Could you check a few things on this model? Use its own coordinates, in mm. A direction names the side the tool comes from. Coordinates: 2 decimals unless noted, no trailing zeros. Write each loop counter-clockwise with the first axis right and the second up, starting at its lowest first coordinate (ties: lowest second). Pieces come first, ordered by that corner, then holes.
Item 1: I want a section at B-B on x = -6. Please give me the cut outline in (y, z), then the cut area to 3 significant figures.
Item 2: If I drill on probe 1 along Z at (x, y) = (-15.5, 7.5); probe 2 along X at (y, z) = (2, -18); probe 3 along Z at (x, y) = (11, 4.75), over which ranges is the centre line in solid material (lowest first)?
Item 3: For P1, Ø8, axis at x = -11.5, z = 4.5, coming from the +Y side; P2, Ø1.1, axis at x = 17.5, z = 2.5, coming from the +Y side; P3, Ø5, axis at x = -11.5, z = 18.5, coming from the -Y side, each with a flat end and sliding along its axis, tell me the tip position at first contact or that it passes through.
Item 4: Thinking about a two-plate mould opening in Z: for faces 4 (the flat face through (0, 4, 23.35)), 5 (the flat face through (0, 0, 0)), 6 (the cylindrical face through (-17.407, 5.403, -11.359)), which applies, +Z half, -Z half, draft (parallel to the pull), parting line (faces both ways), or undercut?
Item 5: I want a section at A-A on z = -5. Please give me the cut outline in (x, y), then the cut area to 3 significant figures.
Item 6: Which directions (+Z, -Z, +X, -X, +Y, -Y) give clear straight access to the entire face, cutting with the end or side of a thin tool? Please do faces 1 (the flat face through (-17.4, 4.2, -0.1)), 2 (the flat face through (11.5, 0.6, -21.35)), 3 (the flat face through (8.345, 4, -22)).
Item 7: I want a section at C-C on y = 7.5. Please give me the cut outline in (x, z) (3 decimals), then the cut area to 3 significant figures.
Autodesk Inventor part; units mm, degrees
ref_plane "YZ Plane" through (0, 0, 0) normal (1, 0, 0) x (0, 1, 0)
ref_plane "XZ Plane" through (0, 0, 0) normal (0, 1, 0) x (-1, 0, 0)
ref_plane "XY Plane" through (0, 0, 0) normal (0, 0, 1) x (1, 0, 0)
sketch "Sketch1" plane through (0, 0, 0) normal (0, 1, 0) x (-1, 0, 0)
  line L0 (17.9, -23.35) -> (-17.9, -23.35)
  line L1 (-17.9, -23.35) -> (-17.9, 23.35)
  line L2 (-17.9, 23.35) -> (17.9, 23.35)
  line L3 (17.9, 23.35) -> (17.9, -23.35)
  point P0 (0, 0)
  dimension "d0" = 35.8
  dimension "d1" = 46.7
  dimension "d2" = 23.35
  dimension "d3" = 17.9
extrude "Extrusion1" add sketch "Sketch1" along normal blind 8.2
sketch "Sketch2" plane through (0, 8.2, 0) normal (0, 1, 0) x (1, 0, 0)
  line L0 (-16.8, -22.25) -> (16.8, -22.25)
  line L1 (16.8, -22.25) -> (16.8, 21.35)
  line L2 (16.8, 21.35) -> (-16.8, 21.35)
  line L3 (-16.8, 21.35) -> (-16.8, -22.25)
  line L4 (-17.9, -23.35) -> (17.9, -23.35)
  line L5 (17.9, -23.35) -> (17.9, 23.35)
  line L6 (-17.9, 23.35) -> (-17.9, -23.35)
  line L7 (17.9, 23.35) -> (-17.9, 23.35)
  point P0 (0, 0)
  dimension "d6" = 1.1
  dimension "d7" = 1.1
  dimension "d8" = 1.1
  dimension "d9" = 2
extrude "Extrusion2" cut sketch "Sketch2" against normal blind 7.1 contours L3 L2 L1 L0
sketch "Sketch6" plane through (17.9, 0, 23.35) normal (1, 0, 0) x (0, 0, -1)
  line L0 (1.1, 8.2) -> (44.7, 8.2)
  line L1 (10.85, 8.2) -> (35.85, 8.2)
  line L2 (35.85, 8.2) -> (35.85, 4.2)
  line L3 (35.85, 4.2) -> (10.85, 4.2)
  line L4 (10.85, 4.2) -> (10.85, 8.2)
  line L5 (46.7, 0) -> (46.7, 8.2)
  point P0 (23.35, 0)
  dimension "d34" = 25
  dimension "d35" = 10.85
  dimension "d36" = 4
extrude "Extrusion6" cut sketch "Sketch6" against normal through all
fillet "Fillet2" radius 4 4 edges at (17.35, 4.2, 12.5) (-17.35, 4.2, 12.5) (-17.35, 4.2, -12.5) (17.35, 4.2, -12.5)
sketch "Sketch9" plane through (0, 8.2, 0) normal (0, 1, 0) x (1, 0, 0)
  point P0 (0, 0)
sketch "Sketch10" plane through (0, 8.2, 0) normal (0, 1, 0) x (1, 0, 0)
  line L0 (-16.8, 21.35) -> (16.8, 21.35)
  line L1 (12.55, 21.35) -> (10.55, 21.35)
  line L2 (10.55, 21.35) -> (10.55, 22.35)
  line L3 (10.55, 22.35) -> (12.55, 22.35)
  line L4 (12.55, 22.35) -> (12.55, 21.35)
  line L5 (8.345, 21.35) -> (6.345, 21.35)
  line L6 (6.345, 21.35) -> (6.345, 22.35)
  line L7 (6.345, 22.35) -> (8.345, 22.35)
  line L8 (8.345, 22.35) -> (8.345, 21.35)
  line L9 (17.9, 23.35) -> (-17.9, 23.35)
  line L10 (17.9, 12.5) -> (17.9, 23.35)
  point P0 (0, 0)
  dimension "d51" = 2
  dimension "d52" = 2
  dimension "d53" = 2.205
  dimension "d54" = 1
  dimension "d55" = 5.35
extrude "Extrusion9" cut sketch "Sketch10" against normal through all
sketch "Sketch12" plane through (0, 8.2, 0) normal (0, 1, 0) x (1, 0, 0)
  line L0 (6.345, 22.35) -> (8.345, 22.35)
  line L1 (6.345, 22.35) -> (8.345, 22.35)
  line L2 (8.345, 22.35) -> (8.345, 22.649)
  line L3 (8.345, 22.649) -> (6.345, 22.649)
  line L4 (6.345, 22.649) -> (6.345, 22.35)
  line L5 (10.55, 22.35) -> (12.55, 22.35)
  line L6 (10.55, 22.35) -> (12.5613, 22.35)
  line L7 (12.5613, 22.35) -> (12.5613, 22.649)
  line L8 (12.5613, 22.649) -> (10.55, 22.649)
  line L9 (10.55, 22.649) -> (10.55, 22.35)
  point P0 (0, 0)
extrude "Extrusion11" cut sketch "Sketch12" against normal through all
sketch "Sketch13" plane through (17.9, 0, -23.35) normal (0, 0, -1) x (-1, 0, 0)
  line L0 (7.35, 0) -> (5.35, 0)
  line L1 (7.35, 8.2) -> (7.35, 1.1)
  line L2 (5.35, 0) -> (7.35, 0)
  line L3 (7.35, 0) -> (7.35, 2.5)
  line L4 (7.35, 2.5) -> (5.35, 2.5)
  line L5 (5.35, 2.5) -> (5.35, 0)
  line L6 (11.555, 0) -> (9.555, 0)
  line L7 (11.555, 8.2) -> (11.555, 1.1)
  line L8 (9.555, 0) -> (11.555, 0)
  line L9 (11.555, 0) -> (11.555, 2.5)
  line L10 (11.555, 2.5) -> (9.555, 2.5)
  line L11 (9.555, 2.5) -> (9.555, 0)
  point P0 (17.9, 0)
  dimension "d66" = 2.5
extrude "Extrusion12" cut sketch "Sketch13" against normal up to surface (2 mm away)
sketch "Sketch14" plane through (0, 8.2, 0) normal (0, 1, 0) x (1, 0, 0)
  line L0 (-16.9, 21.45) -> (16.9, 21.45)
  line L1 (16.9, 21.45) -> (16.9, -22.35)
  line L2 (16.9, -22.35) -> (-16.9, -22.35)
  line L3 (-16.9, -22.35) -> (-16.9, 21.45)
  line L4 (16.8, -22.25) -> (-16.8, -22.25)
  line L5 (-16.8, -22.25) -> (-16.8, -12.5)
  line L6 (-16.8, 21.35) -> (6.345, 21.35)
  line L7 (16.8, 21.35) -> (16.8, 12.5)
  point P0 (0, 0)
  dimension "d69" = 0.1
  dimension "d70" = 0.1
  dimension "d71" = 0.1
  dimension "d72" = 0.1
extrude "Extrusion13" cut sketch "Sketch14" against normal up to surface (7.1 mm away)
properties part number "battery-cover"
Response values:
1. outline: (0, -23.35) - (8.2, -23.35) - (8.2, -21.45) - (1.1, -21.45) - (1.1, 22.35) - (8.2, 22.35) - (8.2, 23.35) - (0, 23.35) - close
1. area: 72.0 mm2
2. probe 1: z = -23.35 to -21.45, 22.35 to 23.35
2. probe 2: x = -17.9 to -16.9, 16.9 to 17.9
2. probe 3: z = -23.35 to -22.65, 22.35 to 23.35
3. P1: stops at y = 1.1
3. P2: stops at y = 4.2
3. P3: stops at y = 0
4. face 4: +Z half
4. face 5: draft
4. face 6: undercut
5. outline: (-17.9, 0) - (17.9, 0) - (17.9, 4.2) - (16.9, 4.2) - (16.9, 1.1) - (-16.9, 1.1) - (-16.9, 4.2) - (-17.9, 4.2) - close
5. area: 45.6 mm2
6. face 1: +X, -X, +Y
6. face 2: -Z, +Y, -Y
6. face 3: -Y
7. outline: (-17.9, -23.35) - (17.9, -23.35) - (17.9, -12.438) - (16.9, -12.438) - (16.9, -21.45) - (12.55, -21.45) - (12.55, -22.35) - (12.561, -22.35) - (12.561, -22.649) - (10.55, -22.649) - (10.55, -21.45) - (8.345, -21.45) - (8.345, -22.649) - (6.345, -22.649) - (6.345, -21.45) - (-16.9, -21.45) - (-16.9, -12.438) - (-17.9, -12.438) - close; (-17.9, 12.438) - (-16.9, 12.438) - (-16.9, 22.35) - (16.9, 22.35) - (16.9, 12.438) - (17.9, 12.438) - (17.9, 23.35) - (-17.9, 23.35) - close
7. area: 137 mm2
